```python
from build123d import *

# Parameters (mm, degrees)
BOSS_EXTRUDE1_DEPTH   = 3
BOSS_EXTRUDE2_DEPTH   = 27
BOSS_EXTRUDE2_2_DEPTH = 27
BOSS_EXTRUDE3_DEPTH   = 3
BOSS_EXTRUDE4_DEPTH   = 6.5
SKETCH5_R             = 3.5
CUT_EXTRUDE1_DEPTH    = 72.292294366
SKETCH6_R             = 2.2
CUT_EXTRUDE2_DEPTH    = 57.599469962
SKETCH7_W             = 10
SKETCH7_H             = 6.5
CUT_EXTRUDE3_DEPTH    = 12.644
SKETCH8_R             = 12
SKETCH8_R_2           = 1.5
CUT_EXTRUDE4_DEPTH    = 53.781068917
SKETCH9_R             = 2.2
CUT_EXTRUDE5_DEPTH    = 51.160654262


with BuildPart() as part:
    # Sketch1 → Boss-Extrude1 (new body)
    with BuildSketch(Plane.XY):
        Polygon((-8, 22.25), (-8, 34.894), (8, 34.894), (8, 22.25), (20, 22.25), (20, -22.25), (-20, -22.25), (-20, 22.25), align=None)
    extrude(amount=BOSS_EXTRUDE1_DEPTH)



with BuildPart() as body_2:
    # Sketch2 → Boss-Extrude2 (new body)
    with BuildSketch(Plane(origin=(0, 0, 0), x_dir=(-1, 0, 0), z_dir=(0, 0, -1))):
        Polygon((31.5, 19.25), (21.614, 19.25), (21.614, -8.75), (24.5, -8.75), (24.5, 16.25), (31.5, 16.25), align=None)
    extrude(amount=-BOSS_EXTRUDE2_DEPTH)


with BuildPart() as body_3:
    # Sketch2 → Boss-Extrude2 2 (new body)
    with BuildSketch(Plane(origin=(0, 0, 0), x_dir=(-1, 0, 0), z_dir=(0, 0, -1))):
        Polygon((-31.5, 16.25), (-31.5, 19.25), (-21.614, 19.25), (-21.614, -8.75), (-24.5, -8.75), (-24.5, 16.25), align=None)
    extrude(amount=-BOSS_EXTRUDE2_2_DEPTH)


with BuildPart() as part_1:
    add(part.part)

    add(body_2.part)  # Boss-Extrude3 merges body 2

    add(body_3.part)  # Boss-Extrude3 merges body 3
    # Sketch3 → Boss-Extrude3 (add)
    with BuildSketch(Plane(origin=(0, 0, 0), x_dir=(-1, 0, 0), z_dir=(0, 0, -1))):
        Polygon((-21.614, -8.75), (21.614, -8.75), (21.614, 19.25), (24.5, 19.25), (21.807, 22.25), (-21.807, 22.25), (-24.5, 19.25), (-21.614, 19.25), align=None)
    extrude(amount=-BOSS_EXTRUDE3_DEPTH)

    # Sketch4 → Boss-Extrude4 (add)
    with BuildSketch(Plane.XY.offset(3)):
        Polygon((-24.5, 19.25), (-21.807, 22.25), (-8, 22.25), (-8, 34.894), (8, 34.894), (8, 22.25), (21.807, 22.25), (24.5, 19.25), align=None)
    extrude(amount=BOSS_EXTRUDE4_DEPTH)

    # Sketch5 → Cut-Extrude1 (cut, through all)
    with BuildSketch(Plane(origin=(24.5, 0, 0), x_dir=(0, 0, -1), z_dir=(1, 0, 0))):
        with Locations(Location((-9, 10.25, 0), (0, 0, 90))):
            Circle(SKETCH5_R)
        Polygon((-27, 16.25), (-3, -8.75), (-27, -8.75), align=None)
    extrude(amount=-CUT_EXTRUDE1_DEPTH, mode=Mode.SUBTRACT)

    # Sketch6 → Cut-Extrude2 (cut, through all)
    with BuildSketch(Plane.XZ.offset(-16.25)):
        with Locations(Location((28, 19.5, 0), (0, 0, 270))):
            Circle(SKETCH6_R)
        with Locations(Location((-28, 19.5, 0), (0, 0, 90))):
            Circle(SKETCH6_R)
        Polygon((24.5, 27), (31.5, 27), (31.5, 24.5), align=None)
        Polygon((24.5, 0), (31.5, 14.5), (31.5, 0), align=None)
        Polygon((-31.5, 0), (-24.5, 0), (-31.5, 14.5), align=None)
        Polygon((-31.5, 24.5), (-24.5, 27), (-31.5, 27), align=None)
    extrude(amount=-CUT_EXTRUDE2_DEPTH, mode=Mode.SUBTRACT)

    # Sketch7 → Cut-Extrude3 (cut)
    with BuildSketch(Plane(origin=(0, 34.894, 0), x_dir=(1, 0, 0), z_dir=(0, 1, 0))):
        with Locations((0, -3.25)):
            Rectangle(SKETCH7_W, SKETCH7_H)
    extrude(amount=-CUT_EXTRUDE3_DEPTH, mode=Mode.SUBTRACT)

    # Sketch8 → Cut-Extrude4 (cut, through all)
    with BuildSketch(Plane.XY.offset(3)):
        with Locations((0, -2.25)):
            Circle(SKETCH8_R)
        with Locations((-15.5, 13.25)):
            Circle(SKETCH8_R_2)
        with Locations((15.5, 13.25)):
            Circle(SKETCH8_R_2)
        with Locations((15.5, -17.75)):
            Circle(SKETCH8_R_2)
        with Locations((-15.5, -17.75)):
            Circle(SKETCH8_R_2)
    extrude(amount=-CUT_EXTRUDE4_DEPTH, mode=Mode.SUBTRACT)

    # Sketch9 → Cut-Extrude5 (cut, through all)
    with BuildSketch(Plane.XY.offset(9.5)):
        with Locations((0, 29.2509)):
            Circle(SKETCH9_R)
    extrude(amount=-CUT_EXTRUDE5_DEPTH, mode=Mode.SUBTRACT)


solid = part_1.part
```
Check sheet for the modelled part. Datum: model origin and axes. Units: mm. A direction names the side the tool comes from. Round coordinates to 2 decimals unless told otherwise and drop trailing zeros. Write each loop counter-clockwise with the first axis right and the second up, starting at its lowest first coordinate (ties: lowest second). Pieces come first, ordered by that corner, then holes. Notation, with made-up numbers: M 62,39 L 115,39 A22 ccw 115,64 Z; hole C 48,50 d9. An arc over 180 degrees is marked long. Write item = value, one per line. Start each with the question number.
1. Gauge pin test, flat ends, axial feed: pin 1 (4 mm diameter, centred on x = -22, y = 20, fed in from -Z); pin 2 (5.5 mm diameter, centred on x = 26.5, z = 8.5, fed in from -Y); pin 3 (10.5 mm diameter, centred on y = 27, z = 6, fed in from +X); pin 4 (8 mm diameter, centred on y = 10.25, z = 9, fed in from +X). Record the tip position at first contact, or that the pin passes through.
2. Scan lines: line 1 (Y direction, x = -15.5, z = 1.2); line 2 (Y direction, x = 0, z = 0.75); line 3 (X direction, y = 5, z = 15). Record each from-to range of solid material in increasing order. Write a range as [from, to].
3. Section check A-A, the plane x = -15.5. Record the cut outline in (y, z), then the cut area to 3 significant figures.
4. Section check D-D, the plane y = -17.75. Record the cut outline in (x, z).
5. Section check B-B, the plane y = -2.25. Record the cut outline in (x, z), then the cut area to 3 significant figures.
6. Tool access check on faces 1 (the flat face through (15, 22.25, 5)), 2 (the flat face through (-15, 22.25, 5)), 3 (the flat face through (-24.5, 6, 10)), 4 (the flat face through (-1, 27, 6.5)), 5 (the cylindrical face through (-16.61, -16.74, 1.52)). Record the directions out of +Z, -Z, +X, -X, +Y, -Y that give a thin tool (end or side, any length) a straight path to the whole face; none if there is none.
7. Release check for a two-part mould opening along Y. For faces 6 (the cylindrical face through (14.39, -16.74, 1.52)), 7 (the flat face through (23.077, 3.925, 15.168)), 8 (the flat face through (8, 29, 5)) record: pulls with the +Y half, pulls with the -Y half, needs draft (parallel to the pull), parting line crosses it, or undercut.
8. Section check C-C, the plane x = -28. Record the cut outline in (y, z).
Results found:
q1.pin_1 = 0
q1.pin_2 = -4.99
q1.pin_3 = 22.26
q1.pin_4 = 24.5
q2.line_1 = [-22.25, -19.25], [-16.25, 11.75], [14.75, 22.25]
q2.line_2 = [-22.25, -14.25], [9.75, 22.25]
q2.line_3 = [-24.5, -21.61], [21.61, 24.5]
q3.outline = M -22.25,0 L -19.25,0 L -19.25,3 L -22.25,3 Z; M -16.25,0 L 11.75,0 L 11.75,3 L -16.25,3 Z; M 14.75,0 L 22.25,0 L 22.25,9.5 L 19.25,9.5 L 19.25,3 L 14.75,3 Z
q3.area = 135 mm^2
q4.outline = M -20,0 L -17,0 L -17,3 L -20,3 Z; M -14,0 L 14,0 L 14,3 L -14,3 Z; M 17,0 L 20,0 L 20,3 L 17,3 Z
q5.outline = M -24.5,0 L -12,0 L -12,3 L -21.61,3 L -21.61,9.24 L -24.5,9.24 Z; M 12,0 L 24.5,0 L 24.5,9.24 L 21.61,9.24 L 21.61,3 L 12,3 Z
q5.area = 111 mm^2
q6.face_1 = +Z, -Z, +X, +Y
q6.face_2 = +Z, -Z, -X, +Y
q6.face_3 = +Z, -Z, -X, -Y
q6.face_4 = -Z, +Y
q6.face_5 = +Z, -Z
q7.face_6 = undercut
q7.face_7 = pulls with the -Y half
q7.face_8 = needs draft
q8.outline = M 16.25,7.25 L 19.25,7.25 L 19.25,17.3 L 16.25,17.3 Z; M 16.25,21.7 L 19.25,21.7 L 19.25,25.75 L 16.25,25.75 Z
